```python
from build123d import *

# Parameters (mm, degrees)
SKETCH1_W           = 232
SKETCH1_H           = 170
BOSS_EXTRUDE1_DEPTH = 4
CUT_EXTRUDE4_DEPTH  = 144.864519601
SKETCH6_R           = 1.523418559
CUT_EXTRUDE5_DEPTH  = 144.864519601
SKETCH8_W           = 232
SKETCH8_H           = 5
CUT_EXTRUDE7_DEPTH  = 144.864519601
SKETCH9_R           = 1.6
CUT_EXTRUDE8_DEPTH  = 144.864519601
SKETCH10_R          = 1.75
CUT_EXTRUDE9_DEPTH  = 144.864519601
SKETCH11_W          = 20
SKETCH11_H          = 33
CUT_EXTRUDE10_DEPTH = 144.864519601
SKETCH12_W          = 21
SKETCH12_H          = 21
CUT_EXTRUDE11_DEPTH = 4
CUT_EXTRUDE12_DEPTH = 4
SKETCH14_W          = 192
SKETCH14_H          = 12
CUT_EXTRUDE13_DEPTH = 4


with BuildPart() as part:
    # Sketch1 → Boss-Extrude1 (new body)
    with BuildSketch(Plane.XY):
        Rectangle(SKETCH1_W, SKETCH1_H)
    extrude(amount=BOSS_EXTRUDE1_DEPTH)

    # Sketch5 → Cut-Extrude4 (cut, through all)
    with BuildSketch(Plane.XY.offset(4)):
        with BuildLine():
            Line((-45.739568187, -1.949021099), (-5.739568187, -1.949021099))
            ThreePointArc((-5.739568187, -1.949021099), (8.402567437, 3.908843277), (14.260431813, 18.050978901))
            Line((14.260431813, 18.050978901), (14.260431813, 28.050978901))
            ThreePointArc((14.260431813, 28.050978901), (8.402567437, 42.193114525), (-5.739568187, 48.050978901))
            Line((-5.739568187, 48.050978901), (-45.739568187, 48.050978901))
            ThreePointArc((-45.739568187, 48.050978901), (-59.881703811, 42.193114525), (-65.739568187, 28.050978901))
            Line((-65.739568187, 28.050978901), (-65.739568187, 18.050978901))
            ThreePointArc((-65.739568187, 18.050978901), (-59.881703811, 3.908843277), (-45.739568187, -1.949021099))
        make_face()
    extrude(amount=-CUT_EXTRUDE4_DEPTH, mode=Mode.SUBTRACT)

    # Sketch6 → Cut-Extrude5 (cut, through all)
    with BuildSketch(Plane.XY.offset(4)):
        with Locations((73.46, 18.098600008)):
            Circle(SKETCH6_R)
        with Locations((25.1238, 10.605600008)):
            Circle(SKETCH6_R)
        with Locations((68.581507234, -12.902099992)):
            Circle(SKETCH6_R)
        with Locations((40.565307234, -12.902099992)):
            Circle(SKETCH6_R)
        with Locations((73.46, -64.527599992)):
            Circle(SKETCH6_R)
        with Locations((25.1238, -64.527599992)):
            Circle(SKETCH6_R)
    extrude(amount=-CUT_EXTRUDE5_DEPTH, mode=Mode.SUBTRACT)

    # Sketch8 → Cut-Extrude7 (cut, through all)
    with BuildSketch(Plane.XY.offset(4)):
        with Locations((0, -82.5)):
            Rectangle(SKETCH8_W, SKETCH8_H)
    extrude(amount=-CUT_EXTRUDE7_DEPTH, mode=Mode.SUBTRACT)

    # Sketch9 → Cut-Extrude8 (cut, through all)
    with BuildSketch(Plane(origin=(0, 0, 0), x_dir=(-1, 0, 0), z_dir=(0, 0, -1))):
        with Locations((106, 44)):
            Circle(SKETCH9_R)
        with Locations((-106, 44)):
            Circle(SKETCH9_R)
        with Locations((0, -51.000000508)):
            Circle(SKETCH9_R)
    extrude(amount=-CUT_EXTRUDE8_DEPTH, mode=Mode.SUBTRACT)

    # Sketch10 → Cut-Extrude9 (cut, through all)
    with BuildSketch(Plane.XY.offset(4)):
        with Locations((-92.249999997, -33.300000021)):
            Circle(SKETCH10_R)
        with Locations((-108.499999997, -63.500000021)):
            Circle(SKETCH10_R)
    extrude(amount=-CUT_EXTRUDE9_DEPTH, mode=Mode.SUBTRACT)

    # Sketch11 → Cut-Extrude10 (cut, through all)
    with BuildSketch(Plane.XY.offset(4)):
        with Locations((106, 68.5)):
            Rectangle(SKETCH11_W, SKETCH11_H)
    cut_extrude10 = extrude(amount=-CUT_EXTRUDE10_DEPTH, mode=Mode.SUBTRACT)

    # Mirror1: Cut-Extrude10 across plane
    add(cut_extrude10.mirror(Plane.ZY), mode=Mode.SUBTRACT)

    # Sketch12 → Cut-Extrude11 (cut)
    with BuildSketch(Plane.XY.offset(4)):
        with Locations((0, -69.5)):
            Rectangle(SKETCH12_W, SKETCH12_H)
    extrude(amount=-CUT_EXTRUDE11_DEPTH, mode=Mode.SUBTRACT)

    # Sketch13 → Cut-Extrude12 (cut)
    with BuildSketch(Plane.XY.offset(4)):
        with BuildLine():
            Line((-48.5, -30), (-48.5, -60))
            ThreePointArc((-48.5, -60), (-50.5, -62), (-52.5, -60))
            Line((-52.5, -60), (-52.5, -30))
            ThreePointArc((-52.5, -30), (-50.5, -28), (-48.5, -30))
        make_face()
        with BuildLine():
            Line((46, 54), (76, 54))
            ThreePointArc((76, 54), (78, 52), (76, 50))
            Line((76, 50), (46, 50))
            ThreePointArc((46, 50), (44, 52), (46, 54))
        make_face()
    extrude(amount=-CUT_EXTRUDE12_DEPTH, mode=Mode.SUBTRACT)

    # Sketch14 → Cut-Extrude13 (cut)
    with BuildSketch(Plane.XY.offset(4)):
        with Locations((0, 79)):
            Rectangle(SKETCH14_W, SKETCH14_H)
    extrude(amount=-CUT_EXTRUDE13_DEPTH, mode=Mode.SUBTRACT)


solid = part.part
```
Here's how the part is built. I have some questions about the finished solid (model axes, mm). A direction names the side the tool comes from. Coordinates: 2 decimals unless noted, no trailing zeros. Order: outer loops, then holes, each group sorted by start corner. A loop starts at its lowest first (then second) coordinate and runs counter-clockwise, first axis right, second up.
1) We'd pull the mould along Y, two halves only. Please class faces 3 (the face through (-2, -2, 0)), 4 (the face through (8.246, 3.754, 2.028)): +Y half, -Y half, draft (parallel to the pull), parting line (faces both ways), or undercut.
2) Imagine slicing it at C-C on z = 1.85. State how many separate pieces and enclosed holes the cut face has, and give its area (3 significant figures).
3) Imagine slicing it at B-B on y = 36. List the corners of the cut face in (x, z) for me.
4) Imagine slicing it at A-A on x = -40.5. List the corners of the cut face in (y, z) for me, and give its area (3 significant figures).
5) I need wall thicknesses on line 1 (Y direction, x = 73.46, z = 1.15); line 2 (X direction, y = -47, z = 3.2); line 3 (Y direction, x = 106, z = 1). Which ranges of each line are inside material? Lowest first, please.
6) Which directions (+Z, -Z, +X, -X, +Y, -Y) give clear straight access to the entire face, cutting with the end or side of a thin tool? Please do faces 1 (the face through (-60.04, 4.07, 2.03)), 2 (the face through (-2, -2, 4)).
7) Will these pins go through, and if not, where does the flat tip stop? pin 1 (2 mm diameter, centred on x = -110.5, z = 1.5, fed in from +Y); pin 2 (1 mm diameter, centred on x = 7.5, z = 2, fed in from -Y); pin 3 (2 mm diameter, centred on y = 64, z = 1.5, fed in from -X).
Response values:
1. face 3: draft
1. face 4: undercut
2. separate pieces: 1
2. enclosed holes: 14
2. area: 30,200 mm2
3. outline: (-116, 0) - (-64.09, 0) - (-64.09, 4) - (-116, 4) - close; (12.61, 0) - (116, 0) - (116, 4) - (12.61, 4) - close
4. outline: (-80, 0) - (-1.95, 0) - (-1.95, 4) - (-80, 4) - close; (48.05, 0) - (73, 0) - (73, 4) - (48.05, 4) - close
4. area: 412 mm2
5. line 1: y = -80 to -66.05, -63 to 16.58, 19.62 to 50, 54 to 73
5. line 2: x = -116 to -52.5, -48.5 to 116
5. line 3: y = -80 to 42.4, 45.6 to 52
6. face 1: +Z, -Z
6. face 2: +Z, +X, -X, +Y, -Y
7. pin 1: stops at y = 52
7. pin 2: stops at y = -59
7. pin 3: stops at x = -96
